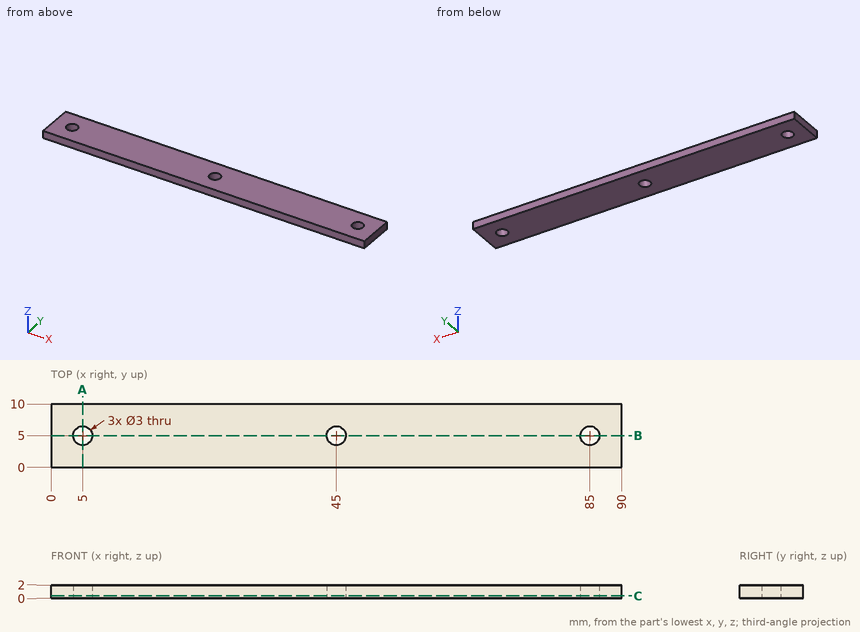
Could you check a few things on this drawing? It's one solid part, dimensions in mm from its lowest x, y, z. Coordinates: 2 decimals unless noted, no trailing zeros. Order: outer loops, then holes, each group sorted by start corner. A loop starts at its lowest first (then second) coordinate and runs counter-clockwise, first axis right, second up.
1. I'm going to push a flat-ended pin straight in: pin 1 (6 mm diameter, centred on x = 33.5, y = 5.5, fed in from -Z). Where does the tip first touch, or does it pass through?
2. If we section it at B-B (y = 5): Please give me the cut outline in (x, z), then the cut area to 3 significant figures.
3. If we section it at A-A (x = 5): Please give me the cut outline in (y, z).
4. If we section it at C-C (z = 0.35): Please give me the cut outline in (x, y), then the cut area to 3 significant figures.
5. I need wall thicknesses on line 1 (X direction, y = 5, z = 0.7); line 2 (X direction, y = 6.25, z = 0.5); line 3 (Y direction, x = 45, z = 0.5). Which ranges of each line are inside material? Lowest first, please.
Entries:
1. pin 1: stops at z = 0
2. outline: (0, 0) - (3.5, 0) - (3.5, 2) - (0, 2) - close; (6.5, 0) - (43.5, 0) - (43.5, 2) - (6.5, 2) - close; (46.5, 0) - (83.5, 0) - (83.5, 2) - (46.5, 2) - close; (86.5, 0) - (90, 0) - (90, 2) - (86.5, 2) - close
2. area: 162 mm2
3. outline: (0, 0) - (3.5, 0) - (3.5, 2) - (0, 2) - close; (6.5, 0) - (10, 0) - (10, 2) - (6.5, 2) - close
4. outline: (0, 0) - (90, 0) - (90, 10) - (0, 10) - close; hole circle Ø3 at (5, 5); hole circle Ø3 at (45, 5); hole circle Ø3 at (85, 5)
4. area: 879 mm2
5. line 1: x = 0 to 3.5, 6.5 to 43.5, 46.5 to 83.5, 86.5 to 90
5. line 2: x = 0 to 4.17, 5.83 to 44.17, 45.83 to 84.17, 85.83 to 90
5. line 3: y = 0 to 3.5, 6.5 to 10
